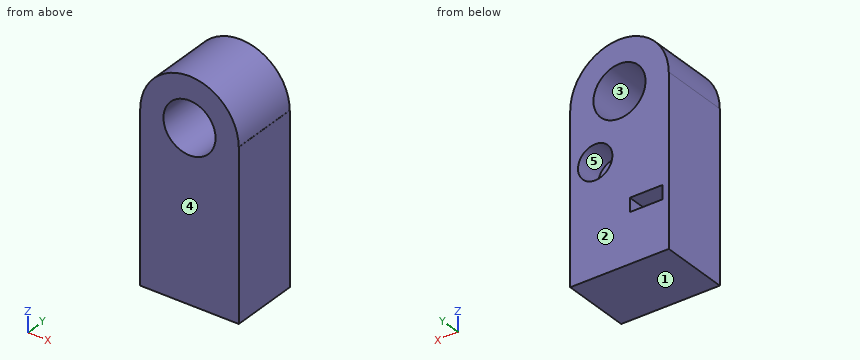
from build123d import *

# Parameters (mm, degrees)
F0_R     = 28.612942
F1_DEPTH = 76.2
F3_W     = 35.79326
F3_H     = 15.010085
F2_R     = 18.912984
F4_DEPTH = 30.226


with BuildPart() as f1:
    # F0 (on Front) → F1 (new body)
    with BuildSketch(Plane.XZ):
        with BuildLine():
            Line((-54.049077, 92.286333), (-54.145753, 92.286333))
            Line((-54.145753, 92.286333), (-54.145753, -92.286333))
            Line((-54.145753, -92.286333), (54.145753, -92.286333))
            Line((54.145753, -92.286333), (54.145753, 92.286333))
            Line((54.145753, 92.286333), (54.049077, 92.286333))
            ThreePointArc((54.049077, 92.286333), (0, 146.335411), (-54.049077, 92.286333))
        make_face()
        with Locations((0, 92.286333)):
            Circle(F0_R, mode=Mode.SUBTRACT)
    extrude(amount=F1_DEPTH)

    # F3 (on Front) + F2 (on Front) → F4 (cut)
    with BuildSketch(Plane.XZ):
        with Locations((-29.298518, -30.562203)):
            Rectangle(F3_W, F3_H)
    with BuildSketch(Plane.XZ):
        with Locations((26.700616, 28.03483)):
            Circle(F2_R)
    extrude(amount=F4_DEPTH, mode=Mode.SUBTRACT)


solid = f1.part
Source: CAD feature listing. Evaluate the final solid. Frame: model axes, mm. Face numbers are marked on the shaded views. A direction names the side the tool comes from. Round coordinates to 2 decimals unless told otherwise and drop trailing zeros. Loops run counter-clockwise (first coordinate to the right, second up) from the corner with the lowest first, then second, coordinate; pieces in that order, holes last.
Q1. Ray query, line 1 (Z direction, x = 0, y = -22); line 2 (X direction, y = -10, z = -25.5); line 3 (Y direction, x = 25.5, z = 41). Return the intervals inside material, ascending.
Q2. Section C-C, the plane z = -32.5. Return loops of the section in (x, y), plus the area to 3 significant figures.
Q3. Section B-B, the plane y = -42. Return loops of the section in (x, z).
Q4. First-contact query: P1, Ø5, axis at x = -5.5, y = -35.5, coming from the +Z side; P2, Ø1, axis at x = 26.5, y = -58.5, coming from the +Z side; P3, Ø5, axis at x = 17.5, y = -53, coming from the +Z side. Flat tips, straight axial feed; report the tip coordinate or a pass-through.
Q5. Access query for the marked faces 4 and 5. Directions: +Z, -Z, +X, -X, +Y, -Y. A direction counts if a zero-diameter tool reaches every point of the face in a straight line with its end or side. Return the directions, or none.
Q6. Section D-D, the plane y = -5.5. Return loops of the section in (x, z), plus the area to 3 significant figures.
Q7. Mould query, pull axis Z, two halves, no side actions, for the marked faces 1, 2 and 3. Classes: pulls with the +Z half, pulls with the -Z half, needs draft (parallel to the pull), parting line crosses it, or undercut.
Q8. Section A-A, the plane x = 0. Return loops of the section in (y, z).
Solutions:
1. line 1: z = -92.29 to 63.67, 120.9 to 146.34
1. line 2: x = -54.15 to -47.2, -11.4 to 54.15
1. line 3: y = -76.2 to -30.23
2. outline: (-54.15, -76.2) - (54.15, -76.2) - (54.15, 0) - (-11.4, 0) - (-11.4, -30.23) - (-47.2, -30.23) - (-47.2, 0) - (-54.15, 0) - close
2. area: 7,170 mm2
3. outline: (-54.15, -92.29) - (54.15, -92.29) - (54.15, 92.29) - (54.05, 92.29) arc R54.05 ccw to (-54.05, 92.29) - (-54.15, 92.29) - close; hole circle Ø57.23 at (0, 92.29)
4. P1: stops at z = 146.25
4. P2: stops at z = 139.67
4. P3: stops at z = 144.21
5. face 4: +Z, -Z, +X, -X, -Y
5. face 5: +Y
6. outline: (-54.15, -92.29) - (54.15, -92.29) - (54.15, 92.29) - (54.05, 92.29) arc R54.05 ccw to (-54.05, 92.29) - (-54.15, 92.29) - close; hole (-47.2, -38.07) - (-11.4, -38.07) - (-11.4, -23.06) - (-47.2, -23.06) - close; hole circle Ø57.23 at (0, 92.29); hole circle Ø37.83 at (26.7, 28.03)
6. area: 20,300 mm2
7. face 1: pulls with the -Z half
7. face 2: needs draft
7. face 3: undercut
8. outline: (-76.2, -92.29) - (0, -92.29) - (0, 63.67) - (-76.2, 63.67) - close; (-76.2, 120.9) - (0, 120.9) - (0, 146.34) - (-76.2, 146.34) - close
